CAD build for the part. Positions are in the model's coordinates, mm. A direction names the side the tool comes from. Give positions to 0.01 mm unless a question says otherwise; leave off trailing zeros. Loops run counter-clockwise (first coordinate to the right, second up) from the corner with the lowest first, then second, coordinate; pieces in that order, holes last. Notation, with made-up numbers: M -21.75,-22.75 L 18.25,-22.75 A13 ccw 18.25,-7.75 Z; hole C 65.5,-31 d5. An arc over 180 degrees is marked long. Answer as CSV lines item,"result".
from build123d import *

# Parameters (mm, degrees)
SKETCH_1_W      = 4
SKETCH_1_H      = 10
EXTRUDE_1_DEPTH = 2


with BuildPart() as part:
    # 草图1 → 凸台-拉伸1 (new, symmetric)
    with BuildSketch(Plane.XY):
        Polygon((-46, 0), (46, 0), (52, 0), (52, 20), (46, 20), (-46, 20), (-52, 20), (-52, 0), align=None)
        with Locations((48, 10)):
            Rectangle(SKETCH_1_W, SKETCH_1_H, mode=Mode.SUBTRACT)
        with Locations((-48, 10)):
            Rectangle(SKETCH_1_W, SKETCH_1_H, mode=Mode.SUBTRACT)
        with Locations((41, 10)):
            Rectangle(SKETCH_1_W, SKETCH_1_H, mode=Mode.SUBTRACT)
        with Locations((-41, 10)):
            Rectangle(SKETCH_1_W, SKETCH_1_H, mode=Mode.SUBTRACT)
    extrude(amount=EXTRUDE_1_DEPTH, both=True)


solid = part.part
1) Band-saw the part on B-B on z = -0.2. Give the cut face in (x, y).
Answer below:
outline,"M -52,0 L 52,0 L 52,20 L -52,20 Z; hole M -50,5 L -46,5 L -46,15 L -50,15 Z; hole M -43,5 L -39,5 L -39,15 L -43,15 Z; hole M 39,5 L 43,5 L 43,15 L 39,15 Z; hole M 46,5 L 50,5 L 50,15 L 46,15 Z"
2) Band-saw the part on A-A on y = 9.25. Give the cut face in (x, z).
Answer below:
outline,"M -52,-2 L -50,-2 L -50,2 L -52,2 Z; M -46,-2 L -43,-2 L -43,2 L -46,2 Z; M -39,-2 L 39,-2 L 39,2 L -39,2 Z; M 43,-2 L 46,-2 L 46,2 L 43,2 Z; M 50,-2 L 52,-2 L 52,2 L 50,2 Z"
3) Drill centre lines: line 1 (X direction, y = 14.5, z = 1.25); line 2 (Y direction, x = -40, z = -0.1). Where is each one in solid material? Low to high. Write a range as from..to.
Answer below:
line 1,"x = -52..-50, -46..-43, -39..39, 43..46, 50..52"
line 2,"y = 0..5, 15..20"
4) Which spindle directions (+Z, -Z, +X, -X, +Y, -Y) get a long thin tool onto all of the face, cutting with end or side? Do faces 1 (the face through (-46, 10, 0)), 2 (the face through (-1, 0, 0)). Say none if no direction does.
Answer below:
face 1,"+Z, -Z"
face 2,"+Z, -Z, +X, -X, -Y"
5) Mould opens along X. For faces 3 (the face through (52, 10, 0)), 4 (the face through (-52, 10, 0)), 5 (the face through (41, 15, 0)) say: +X half, -X half, draft (parallel to the pull), parting line (faces both ways), or undercut.
Answer below:
face 3,"+X half"
face 4,"-X half"
face 5,"undercut"
6) Flat gauge pin, fed straight in: pin 1 (5 mm diameter, centred on x = -40, y = 13, fed in from +Z). Where does the tip first touch, or does it go through?
Answer below:
pin 1,"stops at z = 2"
